Part model, mm, in its own coordinate system. A direction names the side the tool comes from. Give positions to 0.01 mm unless a question says otherwise; leave off trailing zeros. Loops run counter-clockwise (first coordinate to the right, second up) from the corner with the lowest first, then second, coordinate; pieces in that order, holes last. Notation, with made-up numbers: (-2.75, -7) -> (50.25, -7) arc R25 cw to (50.25, 13) -> close; hole circle Ø6 at (30, -31.75). An arc over 180 degrees is marked (long way). One line per question, with ' | ' between items.
```python
from build123d import *

# Parameters (mm, degrees)
BOSS_EXTRUDE1_DEPTH  = 38.1
SHELL1_T             = 5.08
SNAP_START           = -30.286635041
SNAP_HOOK1_DEPTH     = 3.81
MIRROR2_START        = -30.286635041
MIRROR2_COPY_1_DEPTH = 3.81
SKETCH2_W            = 12.7
SKETCH2_H            = 6.35
CUT_EXTRUDE1_DEPTH   = 19.304


# Read off the part's stored shape, not the designer's step: Snap Hook1
with BuildPart() as part:
    # Sketch1 → Boss-Extrude1 (new body)
    with BuildSketch(Plane(origin=(0, 0, 0), x_dir=(1, 0, 0), z_dir=(0, 1, 0))):
        with BuildLine():
            Line((-47.028877551, 32.634950255), (20.916122449, 32.634950255))
            ThreePointArc((20.916122449, 32.634950255), (22.712173673, 31.891001479), (23.456122449, 30.094950255))
            Line((23.456122449, 30.094950255), (23.456122449, -22.864049745))
            ThreePointArc((23.456122449, -22.864049745), (22.712173673, -24.660100969), (20.916122449, -25.404049745))
            Line((20.916122449, -25.404049745), (-47.028877551, -25.404049745))
            ThreePointArc((-47.028877551, -25.404049745), (-48.824928775, -24.660100969), (-49.568877551, -22.864049745))
            Line((-49.568877551, -22.864049745), (-49.568877551, 30.094950255))
            ThreePointArc((-49.568877551, 30.094950255), (-48.824928775, 31.891001479), (-47.028877551, 32.634950255))
        make_face()
    extrude(amount=BOSS_EXTRUDE1_DEPTH)

    # Shell1
    shell1_openings = [part.faces().sort_by_distance(p)[0] for p in [
        (-13.056377551, 38.1, -3.615450255),
    ]]
    offset(amount=SHELL1_T, openings=shell1_openings, kind=Kind.INTERSECTION)

    # Snap Hook1 outline → Snap Hook1 (add)
    with BuildSketch(Plane.YZ.offset(SNAP_START)):
        Polygon((38.998243942, -34.666950255), (42.808243942, -32.634950255), (42.808243942, -30.602950255), (0, -30.602950255), (0, -32.634950255), (38.998243942, -32.634950255), align=None)
    snap_hook1 = extrude(amount=SNAP_HOOK1_DEPTH)

    # Mirror1: Snap Hook1 across plane
    add(snap_hook1.mirror(Plane.XY.offset(-3.615450255)))

    # Mirror2: Snap Hook1 across plane
    add(snap_hook1.mirror(Plane(origin=(-13.056377551, 0, 0), x_dir=(0, 0, 1), z_dir=(1, 0, 0))))

    # Mirror2 copy 1 sketch → Mirror2 copy 1 (add)
    with BuildSketch(Plane(origin=(-26.112755102, 0, -7.23090051), x_dir=(0, 1, 0), z_dir=(-1, 0, 0)).offset(MIRROR2_START)):
        Polygon((38.998243942, -34.666950255), (42.808243942, -32.634950255), (42.808243942, -30.602950255), (0, -30.602950255), (0, -32.634950255), (38.998243942, -32.634950255), align=None)
    extrude(amount=MIRROR2_COPY_1_DEPTH)

    # Sketch2 → Cut-Extrude1 (cut)
    with BuildSketch(Plane(origin=(28.536122449, 0, 0), x_dir=(0, 0, -1), z_dir=(1, 0, 0))):
        with Locations((3.615450255, 10.795)):
            Rectangle(SKETCH2_W, SKETCH2_H)
    extrude(amount=-CUT_EXTRUDE1_DEPTH, mode=Mode.SUBTRACT)


solid = part.part
```
1) Tool access for faces 4 (the flat face through (-28, 22, -30.603)), 5 (the flat face through (-14, 16, -37.715)), 6 (the flat face through (26, 11, -9.965)), 7 (the flat face through (-28, 38.998, 26)), 8 (the cylindrical face through (-52.36, 16.21, 28.31)): list every direction of +Z, -Z, +X, -X, +Y, -Y with a clear straight run to the whole face (end or side of a thin tool).
Found:
face 4: +Y | face 5: -Z, +X, -X, +Y, -Y | face 6: +X | face 7: +Z, +X, -X | face 8: +Z, -X, +Y, -Y
2) Pin check, flat tips, straight feed: P1, Ø0.7, axis at x = -29, y = 38.5, coming from the -Z side; P2, Ø10, axis at x = -13.5, z = -24, coming from the +Y side; P3, Ø4.5, axis at y = 29, z = -32.5, coming from the -X side. Stop position of each tip, or through.
Found:
P1: z = -32.63 | P2: y = 0 | P3: x = -54.65
3) Pull direction Y, two halves, no side cores. Call faces 1 (the flat face through (-28, 38.998, -34)), 2 (the flat face through (2, 42.808, -32)), 3 (the cylindrical face through (26.363, 16.208, 28.193)): pulls with the +Y half, pulls with the -Y half, needs draft (parallel to the pull), parting line crosses it, or undercut.
Found:
face 1: undercut | face 2: pulls with the +Y half | face 3: needs draft
4) Saw through at B-B (z = -27.5). Give the cut face in (x, y), and give its area (3 significant figures).
Found:
outline: (-54.65, -5.08) -> (28.54, -5.08) -> (28.54, 38.1) -> (23.46, 38.1) -> (23.46, 0) -> (-49.57, 0) -> (-49.57, 38.1) -> (-54.65, 38.1) -> close | area: 810 mm2
5) Drill centre lines: line 1 (X direction, y = 8, z = -16.5); line 2 (Z direction, x = -28.5, y = 31); line 3 (Z direction, x = 20, y = 30). Where is each one in solid material? Low to high.
Found:
line 1: -54.65 to -49.57, 23.46 to 28.54 | line 2: -37.71 to -30.6, 23.37 to 30.48 | line 3: -37.71 to -32.63, 25.4 to 30.48
6) Saw through at C-C (x = -21). Give the cut face in (y, z), and give its area (3 significant figures).
Found:
outline: (-5.08, -37.71) -> (38.1, -37.71) -> (38.1, -32.63) -> (0, -32.63) -> (0, 25.4) -> (38.1, 25.4) -> (38.1, 30.48) -> (-5.08, 30.48) -> close | area: 734 mm2
